Model file for the job. Use its own axes, mm. Coordinates: 2 decimals unless noted, no trailing zeros. Order: outer loops, then holes, each group sorted by start corner. A loop starts at its lowest first (then second) coordinate and runs counter-clockwise, first axis right, second up. Notation, with made-up numbers: M 44.25,7.25 L 99.25,7.25 A19 ccw 99.25,42.25 Z; hole C 31.25,-25.75 d2. An arc over 180 degrees is marked long. Return JSON: item names as keys, results as strings.
```python
from build123d import *

# Parameters (mm, degrees)
BOSS_EXTRUDE1_DEPTH = 200
FILLET1_R           = 1
SKETCH2_R           = 1.625
CUT_EXTRUDE1_DEPTH  = 201.249843945
TAP1_D              = 3.242
TAP2_D              = 3.242
SKETCH7_R           = 3.25
CUT_EXTRUDE2_DEPTH  = 186.188120672


with BuildPart() as part:
    # Sketch1 → Boss-Extrude1 (new body)
    with BuildSketch(Plane(origin=(-15, 0, 0), x_dir=(0, 0, -1), z_dir=(1, 0, 0))):
        with BuildLine():
            Line((-8, 6), (-2.2, 6))
            Line((-2.2, 6), (-2.2, 2.5))
            ThreePointArc((-2.2, 2.5), (-4.7, 0), (-2.2, -2.5))
            Line((-2.2, -2.5), (-2.2, -6))
            Line((-2.2, -6), (-8, -6))
            Line((-8, -6), (-8, 6))
        make_face()
    extrude(amount=BOSS_EXTRUDE1_DEPTH)

    # Fillet1
    fillet1_edges = [part.edges().sort_by_distance(p)[0] for p in [
        (85, 6, 8),
        (85, -6, 8),
    ]]
    fillet(fillet1_edges, radius=FILLET1_R)

    # Sketch2 → Cut-Extrude1 (cut, through all)
    with BuildSketch(Plane(origin=(-15, 0, 0), x_dir=(0, 0, -1), z_dir=(1, 0, 0))):
        with Locations((-4.7, 6.75)):
            Circle(SKETCH2_R)
        with Locations((-4.7, -6.75)):
            Circle(SKETCH2_R)
    extrude(amount=CUT_EXTRUDE1_DEPTH, mode=Mode.SUBTRACT)

    # Tap1 (through all)
    with Locations(Plane.XY.offset(8)):
        with Locations((0, 0), (170, 0)):
            Hole(TAP1_D / 2)

    # Tap2 (through all)
    with Locations(Plane.XY.offset(8)):
        with Locations((85, 0)):
            Hole(TAP2_D / 2)

    # Sketch7 → Cut-Extrude2 (cut, through all)
    with BuildSketch(Plane.XY.offset(8)):
        with Locations((120, 0)):
            Circle(SKETCH7_R)
    extrude(amount=-CUT_EXTRUDE2_DEPTH, mode=Mode.SUBTRACT)


solid = part.part
```
Item 1: Wall check: line 1 (X direction, y = 0, z = 5.65); line 2 (Y direction, x = 170, z = 6.3); line 3 (Y direction, x = 72.5, z = 2.5). Give the ranges that are in metal, low to high.
Check result:
{"line 1": "x = -15 to -1.62, 1.62 to 83.38, 86.62 to 116.75, 123.25 to 168.38, 171.62 to 185", "line 2": "y = -6 to -1.62, 1.62 to 6", "line 3": "y = -6 to -2.48, 2.48 to 6"}
Item 2: Saw through at C-C (x = 155.5). Write the cut outline in (y, z) (3 decimals).
Check result:
{"outline": "M -6,2.2 L -2.5,2.2 A2.5 cw 2.5,2.2 L 6,2.2 L 6,3.258 A1.625 cw 6,6.142 L 6,7 A1 ccw 5,8 L -5,8 A1 ccw -6,7 L -6,6.142 A1.625 cw -6,3.258 Z"}
Item 3: Saw through at B-B (x = 120). Write the cut outline in (y, z) (3 decimals), and give its area (3 significant figures).
Check result:
{"outline": "M -6,2.2 L -3.25,2.2 L -3.25,8 L -5,8 A1 ccw -6,7 L -6,6.142 A1.625 cw -6,3.258 Z; M 3.25,2.2 L 6,2.2 L 6,3.258 A1.625 cw 6,6.142 L 6,7 A1 ccw 5,8 L 3.25,8 Z", "area": "27.9 mm2"}
Item 4: Saw through at A-A (y = 0). Write the cut outline in (x, z), and give its area (3 significant figures).
Check result:
{"outline": "M -15,4.7 L -1.62,4.7 L -1.62,8 L -15,8 Z; M 1.62,4.7 L 83.38,4.7 L 83.38,8 L 1.62,8 Z; M 86.62,4.7 L 116.75,4.7 L 116.75,8 L 86.62,8 Z; M 123.25,4.7 L 168.38,4.7 L 168.38,8 L 123.25,8 Z; M 171.62,4.7 L 185,4.7 L 185,8 L 171.62,8 Z", "area": "606 mm2"}
